from build123d import *

# Parameters (mm, degrees)
BOSS_EXTRUDE1_DEPTH = 4
BOSS_EXTRUDE2_DEPTH = 2.5
CUT_EXTRUDE1_DEPTH  = 2.5
CUT_EXTRUDE2_DEPTH  = 7.5
SKETCH5_R           = 1.7
CUT_EXTRUDE3_DEPTH  = 5
SKETCH7_OUTSIDE_W   = 218.062
SKETCH7_OUTSIDE_H   = 108.062
CUT_EXTRUDE4_DEPTH  = 7.5
CUT_EXTRUDE4_TAPER  = 45


with BuildPart() as part:
    # Sketch1 → Boss-Extrude1 (new body)
    with BuildSketch(Plane.XY):
        with BuildLine():
            Line((-35, 28), (75, 28))
            ThreePointArc((75, 28), (103, 0), (75, -28))
            Line((75, -28), (-35, -28))
            ThreePointArc((-35, -28), (-63, 0), (-35, 28))
        make_face()
    extrude(amount=BOSS_EXTRUDE1_DEPTH)

    # Sketch2 → Boss-Extrude2 (add)
    with BuildSketch(Plane(origin=(0, 0, 0), x_dir=(-1, 0, 0), z_dir=(0, 0, -1))):
        with BuildLine():
            Line((-7.348469228, -6), (7.348469228, -6))
            ThreePointArc((7.348469228, -6), (8.737199378, -6.93305329), (8.398250547, -8.571428571))
            ThreePointArc((8.398250547, -8.571428571), (0, -12), (-8.398250547, -8.571428571))
            ThreePointArc((-8.398250547, -8.571428571), (-8.737199378, -6.93305329), (-7.348469228, -6))
        make_face()
        with BuildLine():
            Line((7.348469228, 6), (-7.348469228, 6))
            ThreePointArc((-7.348469228, 6), (-8.737199378, 6.93305329), (-8.398250547, 8.571428571))
            ThreePointArc((-8.398250547, 8.571428571), (0, 12), (8.398250547, 8.571428571))
            ThreePointArc((8.398250547, 8.571428571), (8.737199378, 6.93305329), (7.348469228, 6))
        make_face()
        with BuildLine():
            Line((-47.348469228, 6), (-32.651530772, 6))
            ThreePointArc((-32.651530772, 6), (-31.262800622, 6.93305329), (-31.601749453, 8.571428571))
            ThreePointArc((-31.601749453, 8.571428571), (-40, 12), (-48.398250547, 8.571428571))
            ThreePointArc((-48.398250547, 8.571428571), (-48.737199378, 6.93305329), (-47.348469228, 6))
        make_face()
        with BuildLine():
            Line((-32.651530772, -6), (-47.348469228, -6))
            ThreePointArc((-47.348469228, -6), (-48.737199378, -6.93305329), (-48.398250547, -8.571428571))
            ThreePointArc((-48.398250547, -8.571428571), (-40, -12), (-31.601749453, -8.571428571))
            ThreePointArc((-31.601749453, -8.571428571), (-31.262800622, -6.93305329), (-32.651530772, -6))
        make_face()
    extrude(amount=BOSS_EXTRUDE2_DEPTH)

    # Sketch3 → Cut-Extrude1 (cut)
    with BuildSketch(Plane.XY.offset(4)):
        with BuildLine():
            Line((-17.5, 4.75), (-17.5, -4.75))
            ThreePointArc((-17.5, -4.75), (-17.060660172, -5.810660172), (-16, -6.25))
            Line((-16, -6.25), (-13.765564437, -6.25))
            ThreePointArc((-13.765564437, -6.25), (-13.483765285, -6.290526583), (-13.224806846, -6.408821525))
            Line((-13.224806846, -6.408821525), (-10.218918256, -8.341178475))
            ThreePointArc((-10.218918256, -8.341178475), (-9.959959817, -8.459473417), (-9.678160664, -8.5))
            Line((-9.678160664, -8.5), (9.734435563, -8.5))
            ThreePointArc((9.734435563, -8.5), (10.018134319, -8.458913456), (10.278520672, -8.339030031))
            Line((10.278520672, -8.339030031), (13.251769281, -6.410969969))
            ThreePointArc((13.251769281, -6.410969969), (13.512155635, -6.291086544), (13.795854391, -6.25))
            Line((13.795854391, -6.25), (16, -6.25))
            ThreePointArc((16, -6.25), (17.060660172, -5.810660172), (17.5, -4.75))
            Line((17.5, -4.75), (17.5, 4.75))
            ThreePointArc((17.5, 4.75), (17.060660172, 5.810660172), (16, 6.25))
            Line((16, 6.25), (13.793701886, 6.25))
            ThreePointArc((13.793701886, 6.25), (13.511902734, 6.290526583), (13.252944295, 6.408821525))
            Line((13.252944295, 6.408821525), (10.247055705, 8.341178475))
            ThreePointArc((10.247055705, 8.341178475), (9.988097266, 8.459473417), (9.706298114, 8.5))
            Line((9.706298114, 8.5), (-9.704145609, 8.5))
            ThreePointArc((-9.704145609, 8.5), (-9.987844365, 8.458913456), (-10.248230719, 8.339030031))
            Line((-10.248230719, 8.339030031), (-13.221479328, 6.410969969))
            ThreePointArc((-13.221479328, 6.410969969), (-13.481865681, 6.291086544), (-13.765564437, 6.25))
            Line((-13.765564437, 6.25), (-16, 6.25))
            ThreePointArc((-16, 6.25), (-17.060660172, 5.810660172), (-17.5, 4.75))
        make_face()
        with BuildLine():
            Line((22.5, 4.75), (22.5, -4.75))
            ThreePointArc((22.5, -4.75), (22.939339828, -5.810660172), (24, -6.25))
            Line((24, -6.25), (26.234435563, -6.25))
            ThreePointArc((26.234435563, -6.25), (26.516234715, -6.290526583), (26.775193154, -6.408821525))
            Line((26.775193154, -6.408821525), (29.781081744, -8.341178475))
            ThreePointArc((29.781081744, -8.341178475), (30.040040183, -8.459473417), (30.321839336, -8.5))
            Line((30.321839336, -8.5), (49.734435563, -8.5))
            ThreePointArc((49.734435563, -8.5), (50.018134319, -8.458913456), (50.278520672, -8.339030031))
            Line((50.278520672, -8.339030031), (53.251769281, -6.410969969))
            ThreePointArc((53.251769281, -6.410969969), (53.512155635, -6.291086544), (53.795854391, -6.25))
            Line((53.795854391, -6.25), (56, -6.25))
            ThreePointArc((56, -6.25), (57.060660172, -5.810660172), (57.5, -4.75))
            Line((57.5, -4.75), (57.5, 4.75))
            ThreePointArc((57.5, 4.75), (57.060660172, 5.810660172), (56, 6.25))
            Line((56, 6.25), (53.793701886, 6.25))
            ThreePointArc((53.793701886, 6.25), (53.511902734, 6.290526583), (53.252944295, 6.408821525))
            Line((53.252944295, 6.408821525), (50.247055705, 8.341178475))
            ThreePointArc((50.247055705, 8.341178475), (49.988097266, 8.459473417), (49.706298114, 8.5))
            Line((49.706298114, 8.5), (30.295854391, 8.5))
            ThreePointArc((30.295854391, 8.5), (30.012155635, 8.458913456), (29.751769281, 8.339030031))
            Line((29.751769281, 8.339030031), (26.778520672, 6.410969969))
            ThreePointArc((26.778520672, 6.410969969), (26.518134319, 6.291086544), (26.234435563, 6.25))
            Line((26.234435563, 6.25), (24, 6.25))
            ThreePointArc((24, 6.25), (22.939339828, 5.810660172), (22.5, 4.75))
        make_face()
    extrude(amount=-CUT_EXTRUDE1_DEPTH, mode=Mode.SUBTRACT)

    # Sketch4 → Cut-Extrude2 (cut, through all)
    with BuildSketch(Plane(origin=(0, 0, -2.5), x_dir=(-1, 0, 0), z_dir=(0, 0, -1))):
        with BuildLine():
            Line((-6.5, -6), (8.5, -6))
            ThreePointArc((8.5, -6), (9.207106781, -5.707106781), (9.5, -5))
            Line((9.5, -5), (9.5, 5))
            ThreePointArc((9.5, 5), (9.207106781, 5.707106781), (8.5, 6))
            Line((8.5, 6), (-6.5, 6))
            ThreePointArc((-6.5, 6), (-8.621320344, 5.121320344), (-9.5, 3))
            Line((-9.5, 3), (-9.5, -3))
            ThreePointArc((-9.5, -3), (-8.621320344, -5.121320344), (-6.5, -6))
        make_face()
        with BuildLine():
            Line((-46.5, 6), (-31.5, 6))
            ThreePointArc((-31.5, 6), (-30.792893219, 5.707106781), (-30.5, 5))
            Line((-30.5, 5), (-30.5, -5))
            ThreePointArc((-30.5, -5), (-30.792893219, -5.707106781), (-31.5, -6))
            Line((-31.5, -6), (-46.5, -6))
            ThreePointArc((-46.5, -6), (-48.621320344, -5.121320344), (-49.5, -3))
            Line((-49.5, -3), (-49.5, 3))
            ThreePointArc((-49.5, 3), (-48.621320344, 5.121320344), (-46.5, 6))
        make_face()
    extrude(amount=-CUT_EXTRUDE2_DEPTH, mode=Mode.SUBTRACT)

    # Sketch5 → Cut-Extrude3 (cut, through all)
    with BuildSketch(Plane.XY.offset(1.5)):
        with Locations((-12.5, 0)):
            Circle(SKETCH5_R)
        with Locations((12.5, 0)):
            Circle(SKETCH5_R)
        with Locations((27.5, 0)):
            Circle(SKETCH5_R)
        with Locations((52.5, 0)):
            Circle(SKETCH5_R)
    extrude(amount=-CUT_EXTRUDE3_DEPTH, mode=Mode.SUBTRACT)

    # Sketch7 outside → Cut-Extrude4 (cut, through all)
    with BuildSketch(Plane.XY.offset(4)):
        with Locations((20, 0)):
            Rectangle(SKETCH7_OUTSIDE_W, SKETCH7_OUTSIDE_H)
        Polygon((-35, 22), (-54.052558883, 11), (-54.052558883, -11), (-35, -22), (75, -22), (94.052558883, -11), (94.052558883, 11), (75, 22), align=None, mode=Mode.SUBTRACT)
    extrude(amount=-CUT_EXTRUDE4_DEPTH, taper=CUT_EXTRUDE4_TAPER, mode=Mode.SUBTRACT)


solid = part.part
Geometry: final body of the model. Coordinates: model frame, mm. A direction names the side the tool comes from. Give positions to 0.01 mm unless a question says otherwise; leave off trailing zeros. Order: outer loops, then holes, each group sorted by start corner. A loop starts at its lowest first (then second) coordinate and runs counter-clockwise, first axis right, second up. Notation, with made-up numbers: (-6, 14.25) -> (45, 14.25) arc R27 ccw to (45, 52.25) -> close; hole circle Ø1 at (41.25, -2). An arc over 180 degrees is marked (long way). Put each result on its own line as item: value.
Q1. Reachability of faces 4 (the face through (0, 12, -1)), 5 (the face through (51.74, -7.39, 2.77)), 6 (the face through (-8.75, 6.96, -1.23)) from +Z, -Z, +X, -X, +Y, -Y: full face, straight path, thin tool, end or side. Return the list, or none.
Here are the results:
face 4: -Z, +Y
face 5: +Z
face 6: -Z, -X
Q2. Pin query (flat end, axial travel): pin 1 (1.5 mm diameter, centred on y = 16, z = -1.5, fed in from +X); pin 2 (1.8 mm diameter, centred on x = 55, z = 3.5, fed in from +Y); pin 3 (3 mm diameter, centred on y = 1.5, z = 3.5, fed in from +X); pin 4 (3 mm diameter, centred on x = 44.5, z = 3, fed in from -Y). Return the tip coordinate at first contact, or that it passes through.
Here are the results:
pin 1: passes through
pin 2: stops at y = 23.4
pin 3: stops at x = 96.05
pin 4: stops at y = -24.5
Q3. Section B-B, the plane y = 0. Count the separate pieces of the cut face and the enclosed holes in it, then the cut area to 3 significant figures.
Here are the results:
separate pieces: 7
enclosed holes: 0
area: 356 mm^2
Q4. Section A-A, the plane z = -1.5. Return loops of the section in (x, y), then the cut area to 3 significant figures.
Here are the results:
outline: (-8.4, -8.57) arc R12 ccw to (8.4, -8.57) arc R1.5 ccw to (7.35, -6) -> (-7.35, -6) arc R1.5 ccw to start; (-8.4, 8.57) arc R1.5 ccw to (-7.35, 6) -> (7.35, 6) arc R1.5 ccw to (8.4, 8.57) arc R12 ccw to start; (31.6, -8.57) arc R12 ccw to (48.4, -8.57) arc R1.5 ccw to (47.35, -6) -> (32.65, -6) arc R1.5 ccw to start; (31.6, 8.57) arc R1.5 ccw to (32.65, 6) -> (47.35, 6) arc R1.5 ccw to (48.4, 8.57) arc R12 ccw to start
area: 336 mm^2
Q5. Draft query along X for faces 1 (the face through (57.5, 0, 3)), 2 (the face through (48.75, 6.96, -1.23)), 3 (the face through (-8.728, -6.91, -1.232)). Return one class per face: released by +X, released by -X, zero draft, split by the parting line, or undercut.
Here are the results:
face 1: undercut
face 2: released by +X
face 3: released by -X
Q6. Material intervals for L1, parallel to X at y = -2, z = 0.75; L2, parallel to Z at x = -22, y = -7; L3, parallel to Y at x = -12.5, z = 1, sorted ascending.
Here are the results:
L1: x = -57.3 to -9.5, 9.5 to 30.5, 49.5 to 97.3
L2: z = 0 to 4
L3: y = -25 to -1.7, 1.7 to 25
